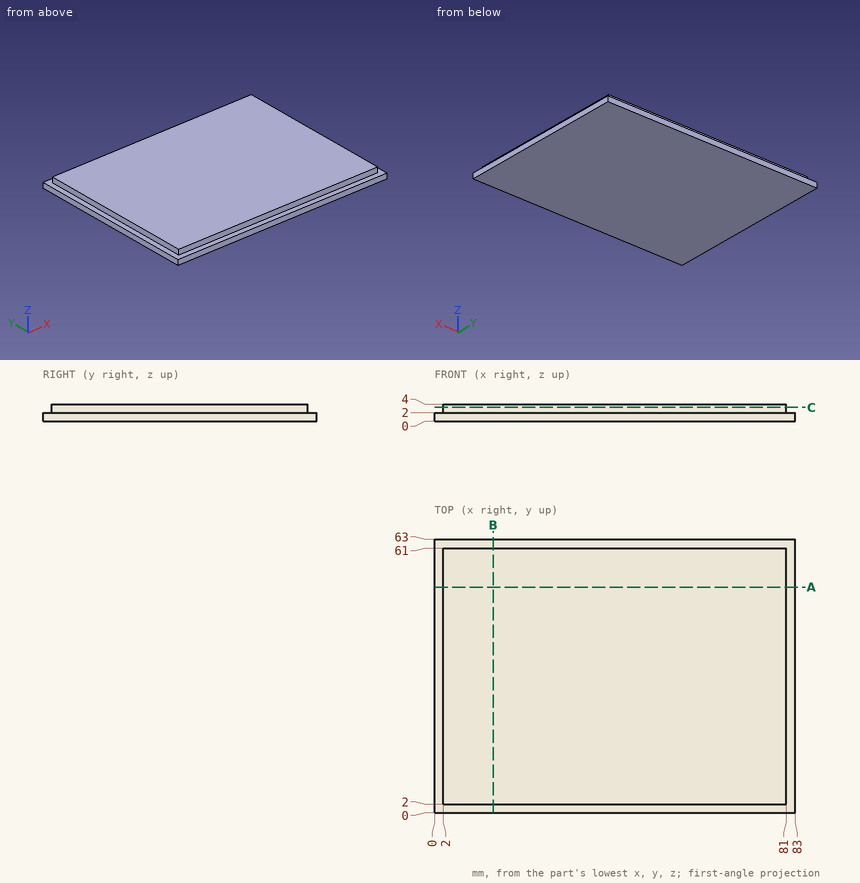
Verification items for this drawing (mm, ordinates from the low corner). Give positions to 0.01 mm unless a question says otherwise; leave off trailing zeros. Order: outer loops, then holes, each group sorted by start corner. A loop starts at its lowest first (then second) coordinate and runs counter-clockwise, first axis right, second up.
1) Cross-section at C-C (z = 3.2). Record the boundary of the cut face in (x, y).
Results are:
outline: (2, 2) - (81, 2) - (81, 61) - (2, 61) - close
2) Gauge pin test, flat ends, axial feed: pin 1 (1 mm diameter, centred on x = 57.5, z = 3.5, fed in from -Y); pin 2 (2 mm diameter, centred on y = 31, z = 3.5, fed in from -X); pin 3 (1 mm diameter, centred on x = 66, z = 3.5, fed in from +Y). Record the tip position at first contact, or that the pin passes through.
Results are:
pin 1: stops at y = 2
pin 2: stops at x = 2
pin 3: stops at y = 61
3) Cross-section at B-B (x = 13.5). Record the boundary of the cut face in (y, z).
Results are:
outline: (0, 0) - (63, 0) - (63, 2) - (61, 2) - (61, 4) - (2, 4) - (2, 2) - (0, 2) - close
4) Material ranges on probe 1 along X at (y, z) = (53, 3.45); probe 2 along Y at (x, z) = (77, 3), recorded low to high.
Results are:
probe 1: x = 2 to 81
probe 2: y = 2 to 61
5) Cross-section at A-A (y = 52). Record the boundary of the cut face in (x, z), then the cut area to 3 significant figures.
Results are:
outline: (0, 0) - (83, 0) - (83, 2) - (81, 2) - (81, 4) - (2, 4) - (2, 2) - (0, 2) - close
area: 324 mm2
